Can you work these out from the model? Positions are in its coordinate system, mm. A direction names the side the tool comes from. Give positions to 0.01 mm unless a question says otherwise; leave off trailing zeros. Order: outer loops, then holes, each group sorted by start corner. A loop starts at its lowest first (then second) coordinate and runs counter-clockwise, first axis right, second up. Notation, with made-up numbers: (71.25, 37.5) -> (100.25, 37.5) arc R20 ccw to (100.25, 57.5) -> close; hole circle Ø9 at (-33, 52.25). An arc over 180 degrees is marked (long way). Answer as a JSON object with one key per item and string values.
```python
from build123d import *

# Parameters (mm, degrees)
BOSS_EXTRU_1_START                          = -25.5
BOSS_EXTRU_1_OUTLINE_R                      = 11.8
BOSS_EXTRU_1_DEPTH                          = 16.5
BOSS_EXTRU_1_START_2                        = -9
BOSS_EXTRU_1_2_DEPTH                        = 14
BOSS_EXTRU_1_3_DEPTH                        = 2
BOSS_EXTRU_1_4_OUTLINE_W                    = 16
BOSS_EXTRU_1_4_OUTLINE_H                    = 9
BOSS_EXTRU_1_4_DEPTH                        = 1.2
BOSS_EXTRU_1_START_3                        = -7.8
BOSS_EXTRU_1_5_DEPTH                        = 7.8
BOSS_EXTRU_1_START_4                        = 2
BOSS_EXTRU_1_6_DEPTH                        = 3
ESQUISSE2_W                                 = 17
ESQUISSE2_H                                 = 9.5
BOSS_EXTRU_2_DEPTH                          = 11.15
ESQUISSE3_W                                 = 2
ESQUISSE3_H                                 = 27.3
BOSS_EXTRU_3_DEPTH                          = 1.236375462
ESQUISSE4_W                                 = 2
ESQUISSE4_H                                 = 27.3
BOSS_EXTRU_4_DEPTH                          = 1.2
ESQUISSE5_W                                 = 26
ESQUISSE5_H                                 = 2
BOSS_EXTRU_5_DEPTH                          = 3.7
ESQUISSE6_W                                 = 15.1
ESQUISSE6_H                                 = 7.6
ENL_V_MAT_EXTRU_1_DEPTH                     = 11.15
ESQUISSE7_W                                 = 14.8
ESQUISSE7_H                                 = 7.3
BOSS_EXTRU_6_DEPTH                          = 11.15
ESQUISSE8_W                                 = 12.7
ESQUISSE8_H                                 = 5.3
ENL_V_MAT_EXTRU_2_DEPTH                     = 9
ESQUISSE9_W                                 = 11
ESQUISSE9_H                                 = 1.5
BOSS_EXTRU_7_DEPTH                          = 9
ESQUISSE10_W                                = 12.2
ESQUISSE10_H                                = 11.3
BOSS_EXTRU_8_DEPTH                          = 10.05
ESQUISSE11_W                                = 8
ESQUISSE11_H                                = 7.7
ENL_V_MAT_EXTRU_3_DEPTH                     = 9
ESQUISSE12_W                                = 5.5
ESQUISSE12_H                                = 3.1
BOSS_EXTRU_9_DEPTH                          = 9
FRAISAGE_POUR_VIS_T_TE_FRAIS_E_M31_AT_COUNT = 2
FRAISAGE_POUR_VIS_T_TE_FRAIS_E_M31_AT_PITCH = 30.61045573
NERVURE1_START                              = -1.5
NERVURE1_OUTLINE_W                          = 3
NERVURE1_OUTLINE_H                          = 9.75
NERVURE1_DEPTH                              = 3
NERVURE2_START                              = -1.5
NERVURE2_OUTLINE_W                          = 3
NERVURE2_OUTLINE_H                          = 9.75
NERVURE2_DEPTH                              = 3
CHANFREIN1_SIZE                             = 2
CONG_4_R                                    = 3.5


with BuildPart() as part:
    # Boss.-Extru.1: read off the stored shape, not the designer's step
    # Boss.-Extru.1 outline → Boss.-Extru.1 (new body)
    with BuildSketch(Plane.XY.offset(BOSS_EXTRU_1_START)):
        Circle(BOSS_EXTRU_1_OUTLINE_R)
    extrude(amount=BOSS_EXTRU_1_DEPTH)

    # Boss.-Extru.1 2 outline → Boss.-Extru.1 2 (add)
    with BuildSketch(Plane.XY.offset(BOSS_EXTRU_1_START_2)):
        with BuildLine():
            ThreePointArc((11.763624538, 0.92581733), (-11.8, 0), (11.763624538, -0.92581733))
            Line((11.763624538, -0.92581733), (11.763624538, 0.92581733))
        make_face()
        with BuildLine():
            Line((-1.55, 10.132127121), (-1.55, 10.890247931))
            ThreePointArc((-1.55, 10.890247931), (0, 11), (1.55, 10.890247931))
            Line((1.55, 10.890247931), (1.55, 10.132127121))
            ThreePointArc((1.55, 10.132127121), (0, -10.25), (-1.55, 10.132127121))
        make_face(mode=Mode.SUBTRACT)
    extrude(amount=BOSS_EXTRU_1_2_DEPTH)

    # Boss.-Extru.1 3 outline → Boss.-Extru.1 3 (add)
    with BuildSketch(Plane.XY):
        with BuildLine():
            Line((2.9e-08, 11.8), (-11.8, 11.8))
            Line((-11.8, 11.8), (-11.8, 0))
            ThreePointArc((-11.8, 0), (-8.343860008, 8.343860028), (2.9e-08, 11.8))
        make_face()
        with BuildLine():
            ThreePointArc((11.763624538, -0.92581733), (-0.463265826, -11.790902628), (-11.8, 0))
            Line((-11.8, 0), (-11.8, -15.5))
            Line((-11.8, -15.5), (11.763624538, -15.5))
            Line((11.763624538, -15.5), (11.763624538, -0.92581733))
        make_face()
        with BuildLine():
            Line((11.763624538, 11.8), (2.9e-08, 11.8))
            ThreePointArc((2.9e-08, 11.8), (8.009848808, 8.665005602), (11.763624538, 0.92581733))
            Line((11.763624538, 0.92581733), (11.763624538, 11.8))
        make_face()
    extrude(amount=BOSS_EXTRU_1_3_DEPTH)

    # Boss.-Extru.1 4 outline → Boss.-Extru.1 4 (add)
    with BuildSketch(Plane.XY.offset(BOSS_EXTRU_1_START_2)):
        with BuildLine():
            Line((11.763624538, 0.92581733), (11.763624538, -0.92581733))
            ThreePointArc((11.763624538, -0.92581733), (11.8, 0), (11.763624538, 0.92581733))
        make_face()
        Rectangle(BOSS_EXTRU_1_4_OUTLINE_W, BOSS_EXTRU_1_4_OUTLINE_H)
    extrude(amount=BOSS_EXTRU_1_4_DEPTH)

    # Boss.-Extru.1 5 outline → Boss.-Extru.1 5 (add)
    with BuildSketch(Plane.XY.offset(BOSS_EXTRU_1_START_3)):
        with BuildLine():
            Line((11.763624538, 0.92581733), (11.763624538, -0.92581733))
            ThreePointArc((11.763624538, -0.92581733), (11.8, 0), (11.763624538, 0.92581733))
        make_face()
    extrude(amount=BOSS_EXTRU_1_5_DEPTH)

    # Boss.-Extru.1 6 outline → Boss.-Extru.1 6 (add)
    with BuildSketch(Plane.XY.offset(BOSS_EXTRU_1_START_4)):
        with BuildLine():
            Line((11.763624538, 0.92581733), (11.763624538, -0.92581733))
            ThreePointArc((11.763624538, -0.92581733), (11.8, 0), (11.763624538, 0.92581733))
        make_face()
    extrude(amount=BOSS_EXTRU_1_6_DEPTH)

    # Esquisse2 → Boss.-Extru.2 (add)
    with BuildSketch(Plane(origin=(0, 0, -7.8), x_dir=(-1, 0, 0), z_dir=(0, 0, -1))):
        Rectangle(ESQUISSE2_W, ESQUISSE2_H)
    extrude(amount=-BOSS_EXTRU_2_DEPTH)

    # Esquisse3 → Boss.-Extru.3 (add)
    with BuildSketch(Plane(origin=(11.763624538, 0, 0), x_dir=(0, 0, -1), z_dir=(1, 0, 0))):
        with Locations((-1, -1.85)):
            Rectangle(ESQUISSE3_W, ESQUISSE3_H)
    extrude(amount=BOSS_EXTRU_3_DEPTH)

    # Esquisse4 → Boss.-Extru.4 (add)
    with BuildSketch(Plane.ZY.offset(11.8)):
        with Locations((1, -1.85)):
            Rectangle(ESQUISSE4_W, ESQUISSE4_H)
    extrude(amount=BOSS_EXTRU_4_DEPTH)

    # Esquisse5 → Boss.-Extru.5 (add)
    with BuildSketch(Plane(origin=(0, 11.8, 0), x_dir=(-1, 0, 0), z_dir=(0, 1, 0))):
        with Locations((0, 1)):
            Rectangle(ESQUISSE5_W, ESQUISSE5_H)
    extrude(amount=BOSS_EXTRU_5_DEPTH)

    # Esquisse6 → Enlèv. mat.-Extru.1 (cut)
    with BuildSketch(Plane.XY.offset(3.35)):
        Rectangle(ESQUISSE6_W, ESQUISSE6_H)
    extrude(amount=-ENL_V_MAT_EXTRU_1_DEPTH, mode=Mode.SUBTRACT)

    # Esquisse7 → Boss.-Extru.6 (add)
    with BuildSketch(Plane.XY.offset(-7.8)):
        Rectangle(ESQUISSE7_W, ESQUISSE7_H)
    extrude(amount=BOSS_EXTRU_6_DEPTH)

    # Esquisse8 → Enlèv. mat.-Extru.2 (cut)
    with BuildSketch(Plane.XY.offset(3.35)):
        Rectangle(ESQUISSE8_W, ESQUISSE8_H)
    extrude(amount=-ENL_V_MAT_EXTRU_2_DEPTH, mode=Mode.SUBTRACT)

    # Esquisse9 → Boss.-Extru.7 (add)
    with BuildSketch(Plane.XY.offset(-5.65)):
        with Locations((0, 1)):
            Rectangle(ESQUISSE9_W, ESQUISSE9_H)
    extrude(amount=BOSS_EXTRU_7_DEPTH)

    # Esquisse10 → Boss.-Extru.8 (add)
    with BuildSketch(Plane(origin=(0, 0, -25.5), x_dir=(-1, 0, 0), z_dir=(0, 0, -1))):
        Rectangle(ESQUISSE10_W, ESQUISSE10_H)
    extrude(amount=BOSS_EXTRU_8_DEPTH)

    # Esquisse11 → Enlèv. mat.-Extru.3 (cut)
    with BuildSketch(Plane(origin=(0, 0, -35.55), x_dir=(-1, 0, 0), z_dir=(0, 0, -1))):
        with Locations((0, 0.35)):
            Rectangle(ESQUISSE11_W, ESQUISSE11_H)
    extrude(amount=-ENL_V_MAT_EXTRU_3_DEPTH, mode=Mode.SUBTRACT)

    # Esquisse12 → Boss.-Extru.9 (add)
    with BuildSketch(Plane(origin=(0, 0, -26.55), x_dir=(-1, 0, 0), z_dir=(0, 0, -1))):
        with Locations((0, 0.35)):
            Rectangle(ESQUISSE12_W, ESQUISSE12_H)
    extrude(amount=BOSS_EXTRU_9_DEPTH)

    # Esquisse13 → Fraisage pour vis à tête fraisée M31 (revolve, cut)
    with BuildSketch(Plane(origin=(-9.5, 12, 2), x_dir=(0, -1, 0), z_dir=(1, 0, 0))):
        Polygon((0, 0), (0, 37.55), (1.6, 37.55), (1.6, 1.599995685), (3, 0.19999191), (3, 0), align=None)
    fraisage_pour_vis_t_te_frais_e_m31 = revolve(axis=Axis((-9.5, 12, 8.35), (0, 0, -1)), mode=Mode.SUBTRACT)

    # Fraisage pour vis à tête fraisée M31 at: Fraisage pour vis à tête fraisée M31 ×2
    with Locations(*[Vector(0.6207029443655612, -0.7840458244617614, 0) * (i * FRAISAGE_POUR_VIS_T_TE_FRAIS_E_M31_AT_PITCH) for i in range(1, FRAISAGE_POUR_VIS_T_TE_FRAIS_E_M31_AT_COUNT)]):
        add(fraisage_pour_vis_t_te_frais_e_m31, mode=Mode.SUBTRACT)

    # Nervure1: read off the stored shape, not the designer's step
    # Nervure1 outline → Nervure1 (add)
    with BuildSketch(Plane.XZ.offset(NERVURE1_START)):
        with Locations((7.6, -30.375)):
            Rectangle(NERVURE1_OUTLINE_W, NERVURE1_OUTLINE_H)
    extrude(amount=NERVURE1_DEPTH)

    # Nervure2: read off the stored shape, not the designer's step
    # Nervure2 outline → Nervure2 (add)
    with BuildSketch(Plane(origin=(0, 0, 0), x_dir=(1, 0, 0), z_dir=(0, 1, 0)).offset(NERVURE2_START)):
        with Locations((-7.6, 30.375)):
            Rectangle(NERVURE2_OUTLINE_W, NERVURE2_OUTLINE_H)
    extrude(amount=NERVURE2_DEPTH)

    # Chanfrein1
    chanfrein1_edges = [part.edges().sort_by_distance(p)[0] for p in [
        (-4, 4.2, -31.05),
        (4, 4.2, -31.05),
    ]]
    chamfer(chanfrein1_edges, length=CHANFREIN1_SIZE)

    # Congé4
    cong_4_edges = [part.edges().sort_by_distance(p)[0] for p in [
        (13, -15.5, 1),
        (-13, -15.5, 1),
        (13, 15.5, 1),
        (-13, 15.5, 1),
    ]]
    fillet(cong_4_edges, radius=CONG_4_R)


solid = part.part
```
1. Will these pins go through, and if not, where does the flat tip stop? pin 1 Ø5 at (x, z) = (2, -29.5) entering from +Y; pin 2 Ø3 at (x, z) = (-3, -32) entering from -Y; pin 3 Ø2.5 at (x, z) = (2, -2.5) entering from +Y.
Worked answers:
{"pin 1": "y = 5.65", "pin 2": "y = -5.65", "pin 3": "y = 11.78"}
2. For faces 4 (the face through (-8, 0, -8)), 5 (the face through (9.1, 0, -30)), 6 (the face through (0, 2.65, -1)), which set-ups out of +Z, -Z, +X, -X, +Y, -Y let a thin tool reach every point of the face, with its end or its side?
Worked answers:
{"face 4": "none", "face 5": "-Z, +X, +Y, -Y", "face 6": "+Z"}
3. Please list where these lines run through material, in increasing order: L1, parallel to X at y = 0, z = -29.5; L2, parallel to X at y = 12, z = 0.35; L3, parallel to X at y = -12, z = 1.95.
Worked answers:
{"L1": "-9.1 to -4, -2.75 to 2.75, 4 to 9.1", "L2": "-13 to -11.1, -7.9 to 13", "L3": "-13 to 6.5, 12.5 to 13"}
4. If we section it at B-B on z = -18: Please give me the cut outline in (x, y), then the cut area to 3 significant figures.
Worked answers:
{"outline": "circle Ø23.6 at (0, 0)", "area": "437 mm²"}
5. If we mould it in two halves opening along X, with no side actions, what happens to faces 1 (the face through (-8, 1.5, -30)), 2 (the face through (11.95, 14.5, 1.01)), 3 (the face through (-8.5, 0, -2))? For each: +X half, -X half, draft (parallel to the pull), parting line (faces both ways), or undercut.
Worked answers:
{"face 1": "draft", "face 2": "+X half", "face 3": "undercut"}
6. If we section it at A-A on z = -2.5: Please give me the cut outline in (x, y).
Worked answers:
{"outline": "circle Ø23.6 at (0, 0); (-8.5, -4.75) -> (8.5, -4.75) -> (8.5, 4.75) -> (-8.5, 4.75) -> close; (-7.4, -3.65) -> (7.4, -3.65) -> (7.4, 3.65) -> (-7.4, 3.65) -> close; (-5.5, 0.25) -> (5.5, 0.25) -> (5.5, 1.75) -> (-5.5, 1.75) -> close; hole (-7.55, -3.8) -> (7.55, -3.8) -> (7.55, 3.8) -> (-7.55, 3.8) -> close; hole (-6.35, -2.65) -> (6.35, -2.65) -> (6.35, 2.65) -> (-6.35, 2.65) -> close; hole (-1.55, 10.13) arc R10.25 ccw (long way) to (1.55, 10.13) -> (1.55, 10.89) arc R11 ccw to (-1.55, 10.89) -> close"}
